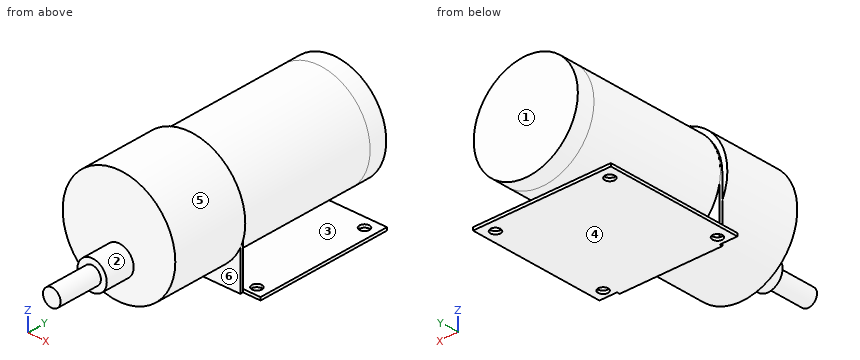
```python
from build123d import *

# Parameters (mm, degrees)
F0_R      = 17.75
F1_DEPTH  = 47
F3_DEPTH  = 1
F4_W      = 47
F4_H      = 1
F5_DEPTH  = 47
F6_R      = 19.2
F7_DEPTH  = 26
F8_R      = 17.75
F9_DEPTH  = 6
F10_R     = 2.99
F11_DEPTH = 25
F12_R     = 5
F13_DEPTH = 10
F15_DEPTH = 1


with BuildPart() as f1:
    # F0 (on Front) → F1 (new body)
    with BuildSketch(Plane.XZ):
        Circle(F0_R)
    extrude(amount=F1_DEPTH)

    # F2 (on face) → F3 (join)
    with BuildSketch(Plane.XZ.offset(47)):
        with BuildLine():
            Line((17.5, -21.25), (17.5, 0))
            ThreePointArc((17.5, 0), (0, 17.5), (-17.5, 0))
            Line((-17.5, 0), (-17.5, -21.25))
            Line((-17.5, -21.25), (17.5, -21.25))
        make_face()
    extrude(amount=F3_DEPTH)

    # F4 (on face) → F5 (join)
    with BuildSketch(Plane(origin=(0, -47, 0), x_dir=(-1, 0, 0), z_dir=(0, 1, 0))):
        with Locations((0, -20.75)):
            Rectangle(F4_W, F4_H)
    extrude(amount=F5_DEPTH)

    # F6 (on face) → F7 (join)
    with BuildSketch(Plane.XZ.offset(48)):
        Circle(F6_R)
    extrude(amount=F7_DEPTH)

    # F8 (on face) → F9 (join)
    with BuildSketch(Plane(origin=(0, 0, 0), x_dir=(-1, 0, 0), z_dir=(0, 1, 0))):
        Circle(F8_R)
    extrude(amount=F9_DEPTH)

    # F10 (on face) → F11 (join)
    with BuildSketch(Plane.XZ.offset(74)):
        with Locations((0, -7.2)):
            Circle(F10_R)
    extrude(amount=F11_DEPTH)

    # F12 (on face) → F13 (join)
    with BuildSketch(Plane.XZ.offset(74)):
        with Locations((0, -7.2)):
            Circle(F12_R)
    extrude(amount=F13_DEPTH)

    # F14 (on face) → F15 (cut, through all)
    with BuildSketch(Plane(origin=(0, 0, -21.25), x_dir=(1, 0, 0), z_dir=(0, 0, -1))):
        with BuildLine():
            ThreePointArc((19.5, 5.7), (18.297918, 5.202082), (17.8, 4))
            Line((17.8, 4), (19.5, 4))
            Line((19.5, 4), (19.5, 5.7))
        make_face()
        with BuildLine():
            Line((19.5, 4), (17.8, 4))
            ThreePointArc((17.8, 4), (19.5, 2.3), (21.2, 4))
            ThreePointArc((21.2, 4), (20.702082, 5.202082), (19.5, 5.7))
            Line((19.5, 5.7), (19.5, 4))
        make_face()
        with BuildLine():
            Line((-19.5, 4), (-17.8, 4))
            ThreePointArc((-17.8, 4), (-18.297918, 5.202082), (-19.5, 5.7))
            Line((-19.5, 5.7), (-19.5, 4))
        make_face()
        with BuildLine():
            ThreePointArc((-19.5, 5.7), (-20.702082, 2.797918), (-17.8, 4))
            Line((-17.8, 4), (-19.5, 4))
            Line((-19.5, 4), (-19.5, 5.7))
        make_face()
        with BuildLine():
            ThreePointArc((21.2, 44), (19.5, 45.7), (17.8, 44))
            Line((17.8, 44), (19.5, 44))
            Line((19.5, 44), (19.5, 42.3))
            ThreePointArc((19.5, 42.3), (20.702082, 42.797918), (21.2, 44))
        make_face()
        with BuildLine():
            Line((-19.5, 44), (-17.8, 44))
            ThreePointArc((-17.8, 44), (-20.702082, 45.202082), (-19.5, 42.3))
            Line((-19.5, 42.3), (-19.5, 44))
        make_face()
        with BuildLine():
            ThreePointArc((-19.5, 42.3), (-18.297918, 42.797918), (-17.8, 44))
            Line((-17.8, 44), (-19.5, 44))
            Line((-19.5, 44), (-19.5, 42.3))
        make_face()
        with BuildLine():
            Line((19.5, 44), (17.8, 44))
            ThreePointArc((17.8, 44), (18.297918, 42.797918), (19.5, 42.3))
            Line((19.5, 42.3), (19.5, 44))
        make_face()
    extrude(amount=-F15_DEPTH, mode=Mode.SUBTRACT)


solid = f1.part
```
Model file for the job. Use its own axes, mm. Face numbers are marked on the shaded views. A direction names the side the tool comes from. Coordinates: 2 decimals unless noted, no trailing zeros. Loops run counter-clockwise (first coordinate to the right, second up) from the corner with the lowest first, then second, coordinate; pieces in that order, holes last. Notation, with made-up numbers: (-7, 78) -> (37, 78) arc R22 cw to (37, 94) -> close; hole circle Ø3 at (70.5, 13). An arc over 180 degrees is marked (long way). Answer as a JSON object with one key per item and string values.
Q1. Cut at D-D (x = 6.5). List the corners of the cut face in (y, z).
Report:
{"outline": "(-74, -18.07) -> (-48, -18.07) -> (-48, -21.25) -> (0, -21.25) -> (0, -20.25) -> (-47, -20.25) -> (-47, -16.52) -> (6, -16.52) -> (6, 16.52) -> (-47, 16.52) -> (-47, 16.25) -> (-48, 16.25) -> (-48, 18.07) -> (-74, 18.07) -> close"}
Q2. Flat gauge pins, fed straight in: P1, Ø10.5, axis at x = -4.5, z = 9, coming from the -Y side; P2, Ø0.5, axis at x = 20.5, z = -20.5, coming from the -Y side; P3, Ø1, axis at y = -35.5, z = -12.5, coming from the -X side; P4, Ø3, axis at x = -19.5, y = -44, coming from the +Z side. Where does each tip first touch, or does it go through?
Report:
{"P1": "stops at y = -74", "P2": "stops at y = -47", "P3": "stops at x = -13.08", "P4": "passes through"}
Q3. 3-axis set-ups, long thin cutter, end or side, ignore diameter. For the marked faces 4, 5 and 6: which of +Z, -Z, +X, -X, +Y, -Y reach the whole face in a straight line?
Report:
{"face 4": "-Z, +X, -X, +Y, -Y", "face 5": "-Y", "face 6": "-Z, -Y"}
Q4. Cut at C-C (z = 4). List the corners of the cut face in (x, y).
Report:
{"outline": "(-18.78, -74) -> (18.78, -74) -> (18.78, -48) -> (17.04, -48) -> (17.04, -47) -> (17.29, -47) -> (17.29, 6) -> (-17.29, 6) -> (-17.29, -47) -> (-17.04, -47) -> (-17.04, -48) -> (-18.78, -48) -> close"}
Q5. Pull direction Z, two halves, no side cores. Call the marked faces 1, 2 and 3: released by +Z, released by -Z, zero draft, split by the parting line, or undercut.
Report:
{"face 1": "zero draft", "face 2": "split by the parting line", "face 3": "undercut"}
Q6. Cut at B-B (x = 0). List the corners of the cut face in (y, z), and give its area (3 significant figures).
Report:
{"outline": "(-99, -10.19) -> (-84, -10.19) -> (-84, -12.2) -> (-74, -12.2) -> (-74, -19.2) -> (-48, -19.2) -> (-48, -21.25) -> (0, -21.25) -> (0, -20.25) -> (-47, -20.25) -> (-47, -17.75) -> (6, -17.75) -> (6, 17.75) -> (-47, 17.75) -> (-47, 17.5) -> (-48, 17.5) -> (-48, 19.2) -> (-74, 19.2) -> (-74, -2.2) -> (-84, -2.2) -> (-84, -4.21) -> (-99, -4.21) -> close", "area": "3,160 mm2"}
Q7. Cut at A-A (y = -7). List the corners of the cut face in (x, z), and give its area (3 significant figures).
Report:
{"outline": "(-23.5, -21.25) -> (23.5, -21.25) -> (23.5, -20.25) -> (-23.5, -20.25) -> close; circle Ø35.5 at (0, 0)", "area": "1,040 mm2"}
Q8. Probe probe 1 along X at (y, z) = (-44, -20.75); probe 2 along Y at (x, z) = (-19.5, -20.5); probe 3 along Z at (x, y) = (-2, -43). List the from-to ranges inside material, lowest first.
Report:
{"probe 1": "x = -23.5 to -21.2, -17.8 to 17.8, 21.2 to 23.5", "probe 2": "y = -47 to -45.7, -42.3 to -5.7, -2.3 to 0", "probe 3": "z = -21.25 to -20.25, -17.64 to 17.64"}
